Autodesk Inventor part; units mm, degrees
ref_plane "YZ Plane" through (0, 0, 0) normal (1, 0, 0) x (0, 1, 0)
ref_plane "XZ Plane" through (0, 0, 0) normal (0, 1, 0) x (-1, 0, 0)
ref_plane "XY Plane" through (0, 0, 0) normal (0, 0, 1) x (1, 0, 0)
sketch "Sketch1" plane through (0, 0, 0) normal (0, 1, 0) x (-1, 0, 0)
  line L0 (-56.25, 58.25) -> (56.25, 58.25)
  line L1 (56.25, 58.25) -> (56.25, -58.25)
  line L2 (56.25, -58.25) -> (-56.25, -58.25)
  line L3 (-56.25, -58.25) -> (-56.25, 58.25)
  line L4 (-56.25, 58.25) -> (56.25, -58.25) construction
  line L5 (56.25, 58.25) -> (-56.25, -58.25) construction
  point P0 (0, 0)
  dimension "d0" = 112.5
  dimension "d1" = 116.5
extrude "Extrusion1" add sketch "Sketch1" along normal blind 3
sketch "Sketch2" plane through (0, 3, 0) normal (0, 1, 0) x (1, 0, 0)
  circle A0 centre (18.5, 28) radius 23.85
  circle A1 centre (37, -23.25) radius 13.85
  circle A2 centre (-35, -40.25) radius 13.85
  circle A3 centre (-30.9, 25.8) radius 13.85
  circle A4 centre (0, -23.25) radius 13.85
  line L0 (56.25, 58.25) -> (-56.25, 58.25)
  line L1 (-56.25, -58.25) -> (56.25, -58.25)
  line L2 (0, -105.9299) -> (0, 123.2086) construction
  line L3 (-76.4777, -40.25) -> (-5.35, -40.25) construction
  line L4 (-123.5447, -23.25) -> (82.5572, -23.25) construction
  line L5 (56.25, -58.25) -> (56.25, 58.25) construction
  point P0 (0, 0)
  dimension "d4" = 47.7
  dimension "d5" = 27.7
  dimension "d6" = 27.7
  dimension "d7" = 27.7
  dimension "d8" = 27.7
  dimension "d9" = 116.5
  dimension "d10" = 112.5
  dimension "d13" = 37
  dimension "d14" = 18.5
  dimension "d15" = 30.9
  dimension "d18" = 18
  dimension "d19" = 35
  dimension "d20" = 35
  dimension "d53" = 28
  dimension "d54" = 25.8
extrude "Extrusion2" cut sketch "Sketch2" against normal blind 5
sketch "Sketch4" plane through (0, 3, 0) normal (0, 1, 0) x (1, 0, 0)
  line L0 (-56.25, 58.25) -> (-56.25, -58.25)
  line L1 (56.25, -58.25) -> (56.25, 58.25)
  line L2 (18.5, -17.4904) -> (18.5, -40.0394) construction
  line L3 (-51.55, 5.4) -> (-51.55, 71.9941) construction
  line L4 (50.75, 5.4) -> (50.75, 69.4565) construction
  line L5 (-73.722, 50) -> (66.5467, 50) construction
  line L6 (66.5467, 30) -> (-76.0779, 30) construction
  circle A0 centre (18.5, 28) radius 23.85
  circle A1 centre (37, -23.25) radius 13.85
  circle A2 centre (-30.9, 25.8) radius 13.85
  circle A3 centre (0, -23.25) radius 13.85
  circle A4 centre (-35, -40.25) radius 13.85
  line L7 (56.25, 58.25) -> (-56.25, 58.25)
  line L8 (-56.25, 58.25) -> (-56.25, -58.25)
  line L9 (-56.25, -58.25) -> (56.25, -58.25)
  line L10 (56.25, -58.25) -> (56.25, 58.25)
  circle A5 centre (-30.9, 25.8) radius 13.85
  circle A6 centre (18.5, 28) radius 23.85
  circle A7 centre (0, -23.25) radius 13.85
  circle A8 centre (37, -23.25) radius 13.85
  circle A9 centre (-35, -40.25) radius 13.85
  line L11 (-56.25, 58.25) -> (-56.25, -58.25)
  line L12 (-56.25, 58.25) -> (-56.25, -58.25)
  line L13 (56.25, -58.25) -> (56.25, 58.25)
  line L14 (56.25, 58.25) -> (56.25, -58.25)
  line L15 (-56.25, 20) -> (-44.75, 20)
  line L16 (-17.05, 20) -> (-5.35, 20)
  line L17 (42.35, 20) -> (56.25, 20)
  line L18 (-56.25, -40.25) -> (-48.85, -40.25)
  circle A10 centre (-35, -40.25) radius 13.85
  circle A11 centre (37, -23.25) radius 13.85
  line L19 (50.85, -23.25) -> (56.25, -23.25)
  circle A12 centre (0, -23.25) radius 13.85
  line L20 (-13.85, -23.25) -> (-13.85, -38.25)
  line L21 (-15.85, -40.25) -> (-21.15, -40.25)
  line L22 (13.85, -23.25) -> (13.85, -31.25)
  line L23 (15.85, -33.25) -> (21.15, -33.25)
  line L24 (23.15, -31.25) -> (23.15, -23.25)
  arc A13 (13.85, -31.25) -> (15.85, -33.25) centre (15.85, -31.25) ccw
  arc A14 (21.15, -33.25) -> (23.15, -31.25) centre (21.15, -31.25) ccw
  arc A15 (-15.85, -40.25) -> (-13.85, -38.25) centre (-15.85, -38.25) ccw
  line L25 (-44.75, 25.8) -> (-44.75, 20)
  circle A16 centre (-30.9, 25.8) radius 13.85
  line L26 (-17.05, 25.8) -> (-17.05, 20)
  line L27 (-5.35, 28) -> (-5.35, 20)
  circle A17 centre (18.5, 28) radius 23.85
  line L28 (42.35, 28) -> (42.35, 20)
  line L29 (-110.6194, 0) -> (115.0669, 0) construction
  line L30 (0, -77.0518) -> (0, 133.3252) construction
  point P0 (-56.25, 17.5733)
  point P1 (-42.0273, 17.5733)
  point P2 (-19.7727, 17.5733)
  point P3 (-2.96, 17.5733)
  point P4 (39.1015, 15.9629)
  point P5 (56.25, 15.9629)
  point P6 (-13.85, -23.25)
  point P7 (-21.15, -40.25)
  point P8 (0, 0)
  point P9 (0, 0)
  point P10 (18.5, -13.25)
  point P11 (18.5, -23.25)
  point P12 (-51.55, 30)
  point P13 (50.75, 50)
  point P14 (50.75, 30)
  point P15 (-13.85, -40.25)
  point P16 (13.85, -33.25)
  point P17 (-56.25, 17.5)
  point P18 (-41.9875, 17.5)
  point P19 (-19.8125, 17.5)
  point P20 (-2.9143, 17.5)
  point P21 (39.1112, 16)
  point P22 (56.25, 16)
  point P23 (-21.15, -40.25)
  point P24 (56.25, 20)
  point P25 (-56.25, 20)
  point P26 (56.25, 0)
  point P27 (-56.25, 0)
  point P28 (-11.2, 39.75)
  dimension "d65" = 27.7
  dimension "d55" = 4.7
  dimension "d56" = 5.5
  dimension "d57" = 13.25
  dimension "d58" = 30
  dimension "d59" = 50
  dimension "d60" = 5.4
  dimension "d61" = 5.4
  dimension "d62" = 18.5
  dimension "d63" = 10
  dimension "d64" = 2
  dimension "d66" = 47.7
  dimension "d67" = 2
  dimension "d68" = 27.7
  dimension "d69" = 23.25
  dimension "d70" = 37
  dimension "d73" = 20
  dimension "d88" = 20
  dimension "d89" = 28
  dimension "d98" = 18.5
  dimension "d99" = 45.05
hole "Hole1" at (-51.55, 3, -30) at (50.75, 3, -50) at (50.75, 3, -30) at (-11.2, 3, -39.75) direction (0, -1, 0) diameter 4.2 end through all
extrude "Extrusion3" cut sketch "Sketch4" against normal blind 10 contours L15 L25 A2 L26 L16 L27 A0 L28 L17 L1 L19 A1 L24 A14 L23 A13 L22 A3 L20 A15 L21 A4 L18 L0 | L18 A4 L21 A15 L20 A3 L22 A13 L23 A14 L24 A1 L19 L1 L9 L0
fillet "Fillet1" radius 2 6 edges at (-56.25, 1.5, -20) (-44.75, 1.5, -20) (-17.05, 1.5, -20) (-5.35, 1.5, -20) (42.35, 1.5, -20) (56.25, 1.5, -20)
sketch "Sketch5" plane through (0, 3, 0) normal (0, 1, 0) x (1, 0, 0)
  line L0 (56.25, 58.25) -> (-56.25, 58.25)
  line L1 (56.25, 58.25) -> (-56.25, 58.25)
  line L2 (-46.75, 25.8) -> (-44.75, 25.8)
  arc A0 (-17.05, 25.8) -> (-44.75, 25.8) centre (-30.9, 25.8) ccw
  arc A1 (-17.05, 25.8) -> (-15.05, 27.8) centre (-17.05, 27.8) ccw
  line L3 (-15.05, 27.8) -> (-15.05, 42.25)
  arc A2 (-13.05, 44.25) -> (-15.05, 42.25) centre (-13.05, 42.25) ccw
  line L4 (-13.05, 44.25) -> (-9.35, 44.25)
  arc A3 (-7.35, 42.25) -> (-9.35, 44.25) centre (-9.35, 42.25) ccw
  line L5 (-7.35, 42.25) -> (-7.35, 29.9796)
  arc A4 (-7.35, 29.9796) -> (-5.35, 27.98) centre (-5.35, 29.98) ccw
  arc A5 (42.35, 27.98) -> (-5.35, 27.98) centre (18.5, 28) ccw
  line L6 (42.35, 27.98) -> (44.35, 27.98)
  line L7 (44.35, 27.98) -> (44.35, 58.25)
  line L8 (44.35, 58.25) -> (-46.75, 58.25)
  line L9 (-46.75, 58.25) -> (-46.75, 25.8)
  line L10 (56.25, 58.25) -> (-56.25, 58.25)
  point P0 (0, 0)
  point P1 (0, 0)
  point P2 (-40.25, 43.25)
  point P3 (-10.75, 52.75)
  point P4 (36.35, 52.75)
  point P5 (54.25, 58.25)
  point P6 (-54.25, 58.25)
  dimension "d75" = 5.5
  dimension "d76" = 5.5
  dimension "d77" = 15
  dimension "d78" = 6.5
  dimension "d79" = 36
  dimension "d80" = 8
hole "Hole2" at (-40.25, 3, -43.25) at (-10.75, 3, -52.75) at (36.35, 3, -52.75) direction (0, -1, 0) diameter 3.2 end through all
sketch "Sketch6" plane through (0, 3, 0) normal (0, 1, 0) x (1, 0, 0)
  line L0 (-73.7148, 40) -> (84.1674, 40) construction
  line L1 (56.25, 58.25) -> (-56.25, 58.25) construction
  arc A0 (-50.25, 36.4) -> (-50.25, 43.6) centre (-50.25, 40) ccw
  arc A1 (50.25, 43.6) -> (50.25, 36.4) centre (50.25, 40) ccw
  line L2 (-56.25, 58.25) -> (-56.25, 22) construction
  line L3 (56.25, 22) -> (56.25, 58.25) construction
  line L4 (-50.25, 43.6) -> (-56.25, 43.6)
  line L5 (-50.25, 36.4) -> (-56.25, 36.4)
  line L6 (50.25, 43.6) -> (56.25, 43.6)
  line L7 (56.25, 22) -> (56.25, 58.25)
  line L8 (50.25, 36.4) -> (56.25, 36.4)
  line L9 (-56.25, 43.6) -> (-56.25, 36.4)
  point P0 (0, 0)
  point P1 (54.25, 58.25)
  point P2 (-54.25, 58.25)
  point P3 (-56.25, 56.25)
  point P4 (56.25, 56.25)
  dimension "d90" = 18.25
  dimension "d91" = 7.2
  dimension "d92" = 7.2
  dimension "d93" = 6
  dimension "d94" = 6
extrude "Extrusion4" cut sketch "Sketch6" against normal blind 10
sketch "Sketch7" plane through (0, 3, 0) normal (0, 1, 0) x (1, 0, 0)
  line L0 (-56.25, 58.25) -> (-56.25, 43.6)
  line L1 (-27.75, 58.25) -> (-56.25, 58.25)
  line L2 (-56.25, 58.25) -> (-56.25, 48.25)
  line L3 (-56.25, 48.25) -> (-27.75, 48.25)
  line L4 (-27.75, 48.25) -> (-27.75, 58.25)
  line L5 (56.25, 58.25) -> (-56.25, 58.25)
  point P0 (0, 0)
  point P1 (-56.25, 56.25)
  point P2 (54.25, 58.25)
  point P3 (-54.25, 58.25)
  point P4 (-56.25, 56.25)
  dimension "d100" = 28.5
  dimension "d101" = 10
extrude "Extrusion5" cut sketch "Sketch7" against normal blind 10
sketch "Sketch8" plane through (56.25, 0, -58.25) normal (0, 0, -1) x (-1, 0, 0)
  line L0 (0, 3) -> (84, 3)
  line L1 (0, 0) -> (84, 0)
  line L2 (84, 3) -> (0, 3)
  line L3 (0, 3) -> (0, 0)
  line L4 (0, 0) -> (84, 0)
  line L5 (84, 0) -> (84, 3)
  point P0 (56.25, 0)
extrude "Extrusion6" cut sketch "Sketch8" against normal blind 0.3
fillet "Fillet3" radius 2 4 edges at (-56.25, 1.5, -48.25) (56.25, 1.5, -57.95) (-27.75, 1.5, -57.95) (-27.75, 1.5, -48.25)
properties part number "Bottle clamping plate 1"
The model under review builds one solid part; all positions refer to its coordinate system, in mm. A direction names the side the tool comes from. Coordinates: 2 decimals unless noted, no trailing zeros. Loops run counter-clockwise (first coordinate to the right, second up) from the corner with the lowest first, then second, coordinate; pieces in that order, holes last. Notation, with made-up numbers: M -15.5,76.5 L 11.5,76.5 A16 cw 11.5,87.5 Z; hole C -11,-3.5 d5. An arc over 180 degrees is marked long. Put each result on its own line as item: value. Start each with the question number.
Q1. Add section D-D (x = 18.5). Write out the cut boundary in (y, z), and give its area (3 significant figures).
Q2. Add section C-C (z = -30). Write out the cut boundary in (x, y), and give its area (3 significant figures).
Q3. Wall thickness on line 1 (Z direction, x = 50.75, y = 1.9); line 2 (Z direction, x = -10.75, y = 0.75); line 3 (X direction, y = 1.4, z = -42): over which ranges is each line inside the solid? List them lowest first.
Q4. For faces 1 (the flat face through (-51, 2, -20)), 2 (the flat face through (-42, 2, -48.25)), 3 (the flat face through (-5.35, 2, -25)), 4 (the flat face through (-53, 2, -36.4)), list the 3-axis set-ups (+Z, -Z, +X, -X, +Y, -Y) from which the entire face can be reached by the end or side of a thin tool; tool diameter is ignored.
Q5. Add section B-B (y = 0.9). Count the separate pieces of the cut face and the enclosed holes in it, and give its area (3 significant figures).
Q6. Add section A-A (x = -51.55). Write out the cut boundary in (y, z), and give its area (4 significant figures).
Q7. Clearance check with flat-ended pins moving along their axes: pin 1 (0.9 mm diameter, centred on x = -54.5, y = 1.5, fed in from -Z); pin 2 (1.5 mm diameter, centred on y = 2, z = -39, fed in from -X). State where each tip first meets the part, or that it passes through.
Q8. The part is to be moulded in two halves that separate along X. For faces 5 (the flat face through (-56.25, 1, -29)), 6 (the flat face through (-17.05, 2, -24)), 7 (the flat face through (1, 3, -47)), say which applies: +X half, -X half, draft (parallel to the pull), parting line (faces both ways), or undercut.
Answers:
1. outline: M 0,-57.95 L 3,-57.95 L 3,-51.85 L 0,-51.85 Z
1. area: 18.3 mm^2
2. outline: M -56.25,0 L -53.65,0 L -53.65,3 L -56.25,3 Z; M -49.45,0 L -44.1,0 L -44.1,3 L -49.45,3 Z; M -17.7,0 L -5.27,0 L -5.27,3 L -17.7,3 Z; M 42.27,0 L 48.65,0 L 48.65,3 L 42.27,3 Z; M 52.85,0 L 56.25,0 L 56.25,3 L 52.85,3 Z
2. area: 90.5 mm^2
3. line 1: z = -57.95 to -52.1, -47.9 to -43.6, -36.4 to -32.1, -27.9 to -20
3. line 2: z = -57.95 to -54.35, -51.15 to -41.8, -37.7 to -20
3. line 3: x = -47.26 to -41.25, -39.25 to -0.81, 37.81 to 47.26
4. face 1: +Z, +X, -X, +Y, -Y
4. face 2: -Z, -X, +Y, -Y
4. face 3: +Z, +Y, -Y
4. face 4: -X, +Y, -Y
5. separate pieces: 1
5. enclosed holes: 7
5. area: 2,040 mm^2
6. outline: M 0,-48.25 L 3,-48.25 L 3,-43.6 L 0,-43.6 Z; M 0,-36.4 L 3,-36.4 L 3,-32.1 L 0,-32.1 Z; M 0,-27.9 L 3,-27.9 L 3,-20 L 0,-20 Z
6. area: 50.55 mm^2
7. pin 1: stops at z = -48.25
7. pin 2: stops at x = -47.1
8. face 5: -X half
8. face 6: undercut
8. face 7: draft
